Model file for the job. Use its own axes, mm. Round coordinates to 2 decimals unless told otherwise and drop trailing zeros. Loops run counter-clockwise (first coordinate to the right, second up) from the corner with the lowest first, then second, coordinate; pieces in that order, holes last. Notation, with made-up numbers: M 32.25,47 L 49.25,47 A7 ccw 49.25,51 Z; hole C 56.5,-0.5 d7. An arc over 180 degrees is marked long. Answer in a Markdown table with one row per item.
from build123d import *

# Parameters (mm, degrees)
BOSS_EXTRUDE2_DEPTH                            = 1.5
CSK_FOR_M3_FLAT_HEAD_MACHINE_SCREW1_AT_2_COUNT = 2
CSK_FOR_M3_FLAT_HEAD_MACHINE_SCREW1_AT_2_PITCH = 177.040281246
CSK_FOR_M3_FLAT_HEAD_MACHINE_SCREW1_AT_3_COUNT = 2
CSK_FOR_M3_FLAT_HEAD_MACHINE_SCREW1_AT_3_PITCH = 203.995944874


with BuildPart() as part:
    # Sketch1 → Boss-Extrude2 (new body)
    with BuildSketch(Plane(origin=(0, 0, 0), x_dir=(1, 0, 0), z_dir=(0, 1, 0))):
        with BuildLine():
            Line((85.023837811, -74.381167696), (143.225208545, -14.836107228))
            ThreePointArc((143.225208545, -14.836107228), (143.81578007, -13.935666345), (144.022845875, -12.878929736))
            Line((144.022845875, -12.878929736), (144.022845875, 95.704196999))
            ThreePointArc((144.022845875, 95.704196999), (143.202744862, 97.684095986), (141.222845875, 98.504196999))
            Line((141.222845875, 98.504196999), (-36.49118484, 98.504196999))
            ThreePointArc((-36.49118484, 98.504196999), (-38.471083828, 97.684095986), (-39.29118484, 95.704196999))
            Line((-39.29118484, 95.704196999), (-39.29118484, 44.391755323))
            ThreePointArc((-39.29118484, 44.391755323), (-39.071891815, 43.305499593), (-38.448362333, 42.389392653))
            Line((-38.448362333, 42.389392653), (81.064297648, -74.426352874))
            ThreePointArc((81.064297648, -74.426352874), (83.053425886, -75.223807903), (85.023837811, -74.381167696))
        make_face()
    extrude(amount=BOSS_EXTRUDE2_DEPTH)

    # Sketch3 → CSK for M3 Flat Head Machine Screw1 (revolve, cut)
    with BuildSketch(Plane(origin=(-35.810496246, 1.5, -94.85013004), x_dir=(0, 0, 1), z_dir=(1, 0, 0))):
        Polygon((0, 0), (0, 1.5), (1.6, 1.5), (1.6, 1.55), (3.15, 0), align=None)
    csk_for_m3_flat_head_machine_screw1 = revolve(axis=Axis((-35.810496246, 7.85, -94.85013004), (0, -1, 0)), mode=Mode.SUBTRACT)

    # CSK for M3 Flat Head Machine Screw1 at 2: CSK for M3 Flat Head Machine Screw1 ×2
    with Locations(*[Vector(0.999998, 0, -0.001999923) * (i * CSK_FOR_M3_FLAT_HEAD_MACHINE_SCREW1_AT_2_PITCH) for i in range(1, CSK_FOR_M3_FLAT_HEAD_MACHINE_SCREW1_AT_2_COUNT)]):
        add(csk_for_m3_flat_head_machine_screw1, mode=Mode.SUBTRACT)

    # CSK for M3 Flat Head Machine Screw1 at 3: CSK for M3 Flat Head Machine Screw1 ×2
    with Locations(*[Vector(0.580964274, 0, 0.813929058) * (i * CSK_FOR_M3_FLAT_HEAD_MACHINE_SCREW1_AT_3_PITCH) for i in range(1, CSK_FOR_M3_FLAT_HEAD_MACHINE_SCREW1_AT_3_COUNT)]):
        add(csk_for_m3_flat_head_machine_screw1, mode=Mode.SUBTRACT)


solid = part.part
1. Saw through at A-A (y = 0.45). Write the cut outline in (x, z).
Verdict:
| item | result |
|---|---|
| outline | M -39.29,-95.7 A2.8 ccw -36.49,-98.5 L 141.22,-98.5 A2.8 ccw 144.02,-95.7 L 144.02,12.88 A2.8 ccw 143.23,14.84 L 85.02,74.38 A2.8 ccw 81.06,74.43 L -38.45,-42.39 A2.8 ccw -39.29,-44.39 Z; hole C -35.81,-94.85 d4.2; hole C 82.7,71.19 d4.2; hole C 141.23,-95.2 d4.2 |
2. Mould opens along Z. For faces 1 (the flat face through (20.47, 0.74, 15.2)), 2 (the flat face through (71, 1.5, -32)) say: +Z half, -Z half, draft (parallel to the pull), parting line (faces both ways), or undercut.
Verdict:
| item | result |
|---|---|
| face 1 | +Z half |
| face 2 | draft |
3. Saw through at B-B (z = 10.5). Write the cut outline in (x, y), and give its area (3 significant figures).
Verdict:
| item | result |
|---|---|
| outline | M 15.66,0 L 144.02,0 L 144.02,1.5 L 15.66,1.5 Z |
| area | 193 mm² |
4. Wall check: probe 1 along Z at (x, y) = (126.5, 1.05); probe 2 along X at (y, z) = (0.85, 5.5); probe 3 along Z at (x, y) = (-18.5, 1.4). Give the ranges that are in metal, low to high.
Verdict:
| item | result |
|---|---|
| probe 1 | z = -98.5 to 31.95 |
| probe 2 | x = 10.55 to 144.02 |
| probe 3 | z = -98.5 to -22.89 |
5. Saw through at C-C (x = 98). Write the cut outline in (y, z).
Verdict:
| item | result |
|---|---|
| outline | M 0,-98.5 L 1.5,-98.5 L 1.5,61.11 L 0,61.11 Z |
